```python
from build123d import *

# Parameters (mm, degrees)
F1_DEPTH = 70
F3_DEPTH = 8
F5_DEPTH = 9


with BuildPart() as f1:
    # F0 (on Right) → F1 (new body)
    with BuildSketch(Plane.YZ):
        Polygon((15.977706, -27.121146), (15.977706, 53.878854), (9.977706, 53.878854), (9.977706, -21.121146), (5.477706, -21.121146), (5.477706, -6.121146), (-0.522294, -6.121146), (-0.522294, -27.121146), align=None)
    extrude(amount=F1_DEPTH)

    # F2 (on face) → F3 (join)
    with BuildSketch(Plane.YZ.offset(70)):
        with BuildLine():
            Line((12.977706, 43.878854), (12.977706, 45.378854))
            ThreePointArc((12.977706, 45.378854), (11.477706, 43.878854), (12.977706, 42.378854))
            Line((12.977706, 42.378854), (12.977706, 43.878854))
        make_face()
        with BuildLine():
            ThreePointArc((12.977706, 42.378854), (14.038366, 42.818193), (14.477706, 43.878854))
            ThreePointArc((14.477706, 43.878854), (14.038366, 44.939514), (12.977706, 45.378854))
            Line((12.977706, 45.378854), (12.977706, 43.878854))
            Line((12.977706, 43.878854), (12.977706, 42.378854))
        make_face()
        with BuildLine():
            Line((12.977706, 23.878854), (12.977706, 25.378854))
            ThreePointArc((12.977706, 25.378854), (11.477706, 23.878854), (12.977706, 22.378854))
            Line((12.977706, 22.378854), (12.977706, 23.878854))
        make_face()
        with BuildLine():
            ThreePointArc((14.477706, 23.878854), (14.038366, 24.939514), (12.977706, 25.378854))
            Line((12.977706, 25.378854), (12.977706, 23.878854))
            Line((12.977706, 23.878854), (12.977706, 22.378854))
            ThreePointArc((12.977706, 22.378854), (14.038366, 22.818193), (14.477706, 23.878854))
        make_face()
        with BuildLine():
            Line((12.977706, 2.878854), (12.977706, 4.378854))
            ThreePointArc((12.977706, 4.378854), (11.477706, 2.878854), (12.977706, 1.378854))
            Line((12.977706, 1.378854), (12.977706, 2.878854))
        make_face()
        with BuildLine():
            ThreePointArc((14.477706, 2.878854), (14.038366, 3.939514), (12.977706, 4.378854))
            Line((12.977706, 4.378854), (12.977706, 2.878854))
            Line((12.977706, 2.878854), (12.977706, 1.378854))
            ThreePointArc((12.977706, 1.378854), (14.038366, 1.818193), (14.477706, 2.878854))
        make_face()
        with BuildLine():
            ThreePointArc((14.477706, -17.121146), (14.038366, -16.060486), (12.977706, -15.621146))
            ThreePointArc((12.977706, -15.621146), (11.917046, -18.181807), (14.477706, -17.121146))
        make_face()
    extrude(amount=F3_DEPTH)

    # F4 (on face) → F5 (cut)
    with BuildSketch(Plane(origin=(0, 0, 0), x_dir=(0, -1, 0), z_dir=(-1, 0, 0))):
        with BuildLine():
            Line((-12.977706, 43.878854), (-12.977706, 45.753854))
            ThreePointArc((-12.977706, 45.753854), (-14.852706, 43.878854), (-12.977706, 42.003854))
            Line((-12.977706, 42.003854), (-12.977706, 43.878854))
        make_face()
        with BuildLine():
            ThreePointArc((-12.977706, 42.003854), (-11.651881, 42.553028), (-11.102706, 43.878854))
            ThreePointArc((-11.102706, 43.878854), (-11.651881, 45.204679), (-12.977706, 45.753854))
            Line((-12.977706, 45.753854), (-12.977706, 43.878854))
            Line((-12.977706, 43.878854), (-12.977706, 42.003854))
        make_face()
        with BuildLine():
            Line((-12.977706, 23.878854), (-12.977706, 25.753854))
            ThreePointArc((-12.977706, 25.753854), (-14.852706, 23.878854), (-12.977706, 22.003854))
            Line((-12.977706, 22.003854), (-12.977706, 23.878854))
        make_face()
        with BuildLine():
            ThreePointArc((-11.102706, 23.878854), (-11.651881, 25.204679), (-12.977706, 25.753854))
            Line((-12.977706, 25.753854), (-12.977706, 23.878854))
            Line((-12.977706, 23.878854), (-12.977706, 22.003854))
            ThreePointArc((-12.977706, 22.003854), (-11.651881, 22.553028), (-11.102706, 23.878854))
        make_face()
        with BuildLine():
            Line((-12.977706, 2.878854), (-12.977706, 4.753854))
            ThreePointArc((-12.977706, 4.753854), (-14.852706, 2.878854), (-12.977706, 1.003854))
            Line((-12.977706, 1.003854), (-12.977706, 2.878854))
        make_face()
        with BuildLine():
            ThreePointArc((-11.102706, 2.878854), (-11.651881, 4.204679), (-12.977706, 4.753854))
            Line((-12.977706, 4.753854), (-12.977706, 2.878854))
            Line((-12.977706, 2.878854), (-12.977706, 1.003854))
            ThreePointArc((-12.977706, 1.003854), (-11.651881, 1.553028), (-11.102706, 2.878854))
        make_face()
        with BuildLine():
            ThreePointArc((-12.977706, -15.246146), (-14.852706, -17.121146), (-12.977706, -18.996146))
            Line((-12.977706, -18.996146), (-12.977706, -17.121146))
            Line((-12.977706, -17.121146), (-12.977706, -15.246146))
        make_face()
        with BuildLine():
            Line((-12.977706, -17.121146), (-12.977706, -18.996146))
            ThreePointArc((-12.977706, -18.996146), (-11.651881, -18.446972), (-11.102706, -17.121146))
            ThreePointArc((-11.102706, -17.121146), (-11.651881, -15.795321), (-12.977706, -15.246146))
            Line((-12.977706, -15.246146), (-12.977706, -17.121146))
        make_face()
    extrude(amount=-F5_DEPTH, mode=Mode.SUBTRACT)


solid = f1.part
```
CAD build for the part. Positions are in the model's coordinates, mm. A direction names the side the tool comes from. Round coordinates to 2 decimals unless told otherwise and drop trailing zeros. Loops run counter-clockwise (first coordinate to the right, second up) from the corner with the lowest first, then second, coordinate; pieces in that order, holes last. Notation, with made-up numbers: M 51,84 L 102,84 A11 cw 102,91 Z; hole C 67,-17.5 d10. An arc over 180 degrees is marked long. Use a Markdown table: item, result. Add a question column.
(1) Drill centre lines: line 1 (Z direction, x = 8.5, y = 13.25); line 2 (X direction, y = 4.25, z = -20.5); line 3 (Y direction, x = 40, z = 5.5). Where is each one in solid material? Low to high.
(2) Cut at D-D (y = 3.75). Give the cut face in (x, z), and give its area (3 significant figures).
(3) Cut at C-C (z = 27). Give the cut face in (x, y).
(4) Cut at A-A (z = -12). Give the cut face in (x, y).
(5) Which spindle directions (+Z, -Z, +X, -X, +Y, -Y) get a long thin tool onto all of the face, cutting with end or side? Do faces 1 (the face through (9, 13, -17)), 2 (the face through (35, 9.978, 17)), 3 (the face through (35, 15.978, 13)). Say none if no direction does.
(6) Flat gauge pins, fed straight in: pin 1 (2 mm diameter, centred on x = 39, z = 31.5, fed in from -Y); pin 2 (3 mm diameter, centred on x = 45, y = 1.5, fed in from +Z); pin 3 (1.1 mm diameter, centred on y = 13.5, z = 2.5, fed in from -X); pin 4 (8 mm diameter, centred on y = 4.5, z = 42.5, fed in from +X). Where does each tip first touch, or does it go through?
(7) Cut at B-B (x = 58). Give the cut face in (y, z).
(8) Pull direction Z, two halves, no side cores. Call faces 4 (the face through (9, 13, 24)), 5 (the face through (35, 3, -6.121)), 6 (the face through (78, 13, -17)): +Z half, -Z half, draft (parallel to the pull), parting line (faces both ways), or undercut.
Geometry says:
| question | item | result |
|---|---|---|
| 1 | line 1 | z = -27.12 to -18.98, -15.27 to 1.02, 4.73 to 22.02, 25.73 to 42.02, 45.73 to 53.88 |
| 1 | line 2 | x = 0 to 70 |
| 1 | line 3 | y = 9.98 to 15.98 |
| 2 | outline | M 0,-27.12 L 70,-27.12 L 70,-6.12 L 0,-6.12 Z |
| 2 | area | 1,470 mm² |
| 3 | outline | M 0,9.98 L 70,9.98 L 70,15.98 L 0,15.98 Z |
| 4 | outline | M 0,-0.52 L 70,-0.52 L 70,5.48 L 0,5.48 Z; M 0,9.98 L 70,9.98 L 70,15.98 L 0,15.98 Z |
| 5 | face 1 | -X |
| 5 | face 2 | +Z, +X, -X |
| 5 | face 3 | +Z, -Z, +X, -X, +Y |
| 6 | pin 1 | stops at y = 9.98 |
| 6 | pin 2 | stops at z = -6.12 |
| 6 | pin 3 | stops at x = 9 |
| 6 | pin 4 | passes through |
| 7 | outline | M -0.52,-27.12 L 15.98,-27.12 L 15.98,53.88 L 9.98,53.88 L 9.98,-21.12 L 5.48,-21.12 L 5.48,-6.12 L -0.52,-6.12 Z |
| 8 | face 4 | undercut |
| 8 | face 5 | +Z half |
| 8 | face 6 | draft |
